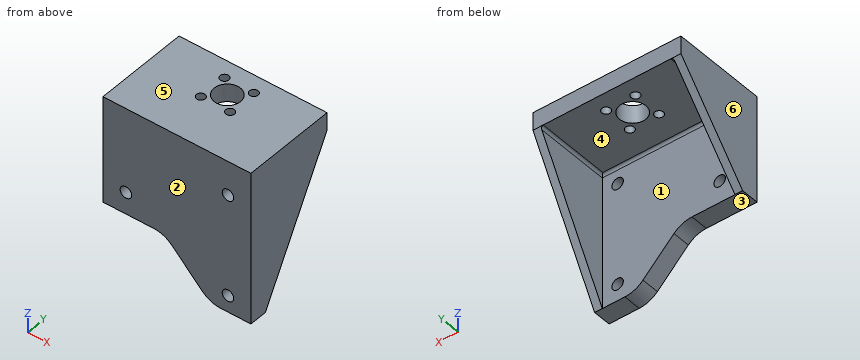
from build123d import *

# Parameters (mm, degrees)
SKETCH1_W            = 58
SKETCH1_H            = 60
BOSS_EXTRUDE1_DEPTH  = 7
SKETCH2_W            = 58
SKETCH2_H            = 7
BOSS_EXTRUDE2_DEPTH  = 30
SKETCH5_R            = 5.15
CUT_EXTRUDE1_DEPTH   = 87.844688957
M3_CLEARANCE_HOLE1_D = 3.4
SUPPORT_DEPTH        = 3
M4_CLEARANCE_HOLE2_D = 4.5
CUT_EXTRUDE5_DEPTH   = 89.67919711
BOSS_EXTRUDE6_DEPTH  = 3
FILLET2_R            = 10
FILLET3_R            = 1


with BuildPart() as part:
    # Sketch1 → Boss-Extrude1 (new body)
    with BuildSketch(Plane(origin=(0, 0, 0), x_dir=(1, 0, 0), z_dir=(0, 1, 0))):
        with Locations((29, 30)):
            Rectangle(SKETCH1_W, SKETCH1_H)
    extrude(amount=BOSS_EXTRUDE1_DEPTH)

    # Sketch2 → Boss-Extrude2 (add)
    with BuildSketch(Plane(origin=(0, 7, 0), x_dir=(1, 0, 0), z_dir=(0, 1, 0))):
        with Locations((29, 3.5)):
            Rectangle(SKETCH2_W, SKETCH2_H)
    extrude(amount=BOSS_EXTRUDE2_DEPTH)

    # Sketch5 → Cut-Extrude1 (cut, through all)
    with BuildSketch(Plane(origin=(0, 0, -7), x_dir=(-1, 0, 0), z_dir=(0, 0, -1))):
        with Locations((-29, 24.5)):
            Circle(SKETCH5_R)
    extrude(amount=-CUT_EXTRUDE1_DEPTH, mode=Mode.SUBTRACT)

    # M3 Clearance Hole1 (through all)
    with Locations(Plane(origin=(0, 0, -7), x_dir=(-1, 0, 0), z_dir=(0, 0, -1))):
        with Locations((-34.75, 18.75), (-23.25, 18.75), (-23.25, 30.25), (-34.75, 30.25)):
            Hole(M3_CLEARANCE_HOLE1_D / 2)

    # Sketch15 → support (add)
    with BuildSketch(Plane(origin=(58, 0, 0), x_dir=(0, 0, -1), z_dir=(1, 0, 0))):
        Polygon((60, 7), (7, 37), (7, 7), align=None)
    extrude(amount=-SUPPORT_DEPTH)

    # M4 Clearance Hole2 (through all)
    with Locations(Plane(origin=(0, 7, 0), x_dir=(1, 0, 0), z_dir=(0, 1, 0))):
        with Locations((49, 53.4), (49, 13.4), (9, 33.4)):
            Hole(M4_CLEARANCE_HOLE2_D / 2)

    # Sketch21 → Cut-Extrude5 (cut, through all)
    with BuildSketch(Plane(origin=(0, 7, 0), x_dir=(1, 0, 0), z_dir=(0, 1, 0))):
        Polygon((42, 60), (24, 42), (0, 42), (0, 60), align=None)
    extrude(amount=-CUT_EXTRUDE5_DEPTH, mode=Mode.SUBTRACT)

    # Sketch22 → Boss-Extrude6 (add)
    with BuildSketch(Plane.ZY):
        Polygon((-42, 7), (-7, 37), (-7, 7), align=None)
    extrude(amount=-BOSS_EXTRUDE6_DEPTH)

    # Fillet2
    fillet2_edges = [part.edges().sort_by_distance(p)[0] for p in [
        (42, 3.5, -60),
        (24, 3.5, -42),
    ]]
    fillet(fillet2_edges, radius=FILLET2_R)

    # Fillet3
    fillet3_edges = [part.edges().sort_by_distance(p)[0] for p in [
        (29, 7, -7),
        (55, 22, -7),
        (3, 22, -7),
    ]]
    fillet(fillet3_edges, radius=FILLET3_R)


solid = part.part
For this review, take the finished solid that the model builds, in its own axes (mm). Face numbers are marked on the shaded views. A direction names the side the tool comes from. Give positions to 0.01 mm unless a question says otherwise; leave off trailing zeros. Order: outer loops, then holes, each group sorted by start corner. A loop starts at its lowest first (then second) coordinate and runs counter-clockwise, first axis right, second up. Notation, with made-up numbers: M 78.25,-12.5 L 88.25,-12.5 A37 cw 88.25,25.5 Z; hole C 19.5,-3.5 d10. An arc over 180 degrees is marked long. Answer in a Markdown table with one row per item. Add a question column.
(1) Consider section C-C on y = 5.5. State the section outline as (x, z) points.
(2) Consider section D-D on z = -4. State the section outline as (x, y) points.
(3) Consider section A-A on x = 29. State the section outline as (y, z) points.
(4) Mouldability with a two-part tool opening along X and no side actions: class the marked faces 4, 5 and 6 as +X half, -X half, draft (parallel to the pull), parting line (faces both ways), or undercut.
(5) Wall thickness on probe 1 along Z at (x, y) = (49, 1.5); probe 2 along Y at (x, z) = (23, -2); probe 3 along X at (y, z) = (18, -4): over which ranges is each line inside the solid? List them lowest first. Write a range as [from, to].
(6) For pin 1 (2 mm diameter, centred on x = 34.5, z = -47, fed in from +Y); pin 2 (3.5 mm diameter, centred on x = 11.5, y = 4.5, fed in from -Z); pin 3 (6 mm diameter, centred on y = 5, z = -43, fed in from -X); pin 4 (4 mm diameter, centred on x = 23.25, y = 18.75, fed in from -Z), all flat-tipped, find the tip position at first contact; note any pin that passes through.
(7) Consider section B-B on z = -13.4. State the section outline as (x, y) points.
(8) For the marked faces 1, 2 and 3, list the 3-axis set-ups (+Z, -Z, +X, -X, +Y, -Y) from which the entire face can be reached by the end or side of a thin tool; tool diameter is ignored.
Evaluation:
| question | item | result |
|---|---|---|
| 1 | outline | M 0,-42 L 19.86,-42 A10 cw 26.93,-44.93 L 39.07,-57.07 A10 ccw 46.14,-60 L 58,-60 L 58,0 L 0,0 Z; hole C 9,-33.4 d4.5; hole C 49,-53.4 d4.5; hole C 49,-13.4 d4.5 |
| 2 | outline | M 0,0 L 58,0 L 58,37 L 0,37 Z; hole C 23.25,18.75 d3.4; hole C 23.25,30.25 d3.4; hole C 29,24.5 d10.3; hole C 34.75,18.75 d3.4; hole C 34.75,30.25 d3.4 |
| 3 | outline | M 0,-47 L 7,-47 L 7,-8 A1 cw 8,-7 L 19.35,-7 L 19.35,0 L 0,0 Z; M 29.65,-7 L 37,-7 L 37,0 L 29.65,0 Z |
| 4 | face 4 | undercut |
| 4 | face 5 | draft |
| 4 | face 6 | -X half |
| 5 | probe 1 | z = [-60, -55.65], [-51.15, -15.65], [-11.15, 0] |
| 5 | probe 2 | y = [0, 17.07], [20.43, 28.57], [31.93, 37] |
| 5 | probe 3 | x = [0, 21.72], [24.78, 33.22], [36.28, 58] |
| 6 | pin 1 | stops at y = 7 |
| 6 | pin 2 | stops at z = -42 |
| 6 | pin 3 | stops at x = 0 |
| 6 | pin 4 | stops at z = -7 |
| 7 | outline | M 0,0 L 46.75,0 L 46.75,7 L 3,7 L 3,31.51 L 0,31.51 Z; M 51.25,0 L 58,0 L 58,33.38 L 55,33.38 L 55,7 L 51.25,7 Z |
| 8 | face 1 | -Z, +Y |
| 8 | face 2 | +Z, -Z, +X, -X, -Y |
| 8 | face 3 | -Z, -X, +Y, -Y |
